from build123d import *

# Parameters (mm, degrees)
BOSS_EXTRUDE1_DEPTH = 5
FILLET3_R           = 1
FILLET4_R           = 1
FILLET5_R           = 4


with BuildPart() as part:
    # Sketch1 → Boss-Extrude1 (new body)
    with BuildSketch(Plane.XY):
        Polygon((0, 5), (0, 19.982808697), (0, 24.6), (0, 29.8), (6.8, 29.8), (6.8, 26.8), (4.8, 26.8), (4.8, 24.6), (10, 24.6), (10, 21.2), (4.8, 21.2), (4.8, 19.6), (20, 19.6), (20, 5), (20, 0), (15, 0), (15, 5), (11.5, 5), (11.5, 8), (12.6, 8), (12.6, 10.3), (11.5, 10.3), (11.5, 15), (8.5, 15), (8.5, 10.3), (7.4, 10.3), (7.4, 8), (8.5, 8), (8.5, 5), (5, 5), (5, 0), (0, 0), align=None)
    extrude(amount=BOSS_EXTRUDE1_DEPTH)

    # Fillet3
    fillet3_edges = [part.edges().sort_by_distance(p)[0] for p in [
        (10, 21.2, 2.5),
        (20, 19.6, 2.5),
    ]]
    fillet(fillet3_edges, radius=FILLET3_R)

    # Fillet4
    fillet4_edges = [part.edges().sort_by_distance(p)[0] for p in [
        (6.8, 29.8, 2.5),
        (6.8, 26.8, 2.5),
        (10, 24.6, 2.5),
    ]]
    fillet(fillet4_edges, radius=FILLET4_R)

    # Fillet5
    fillet5_edges = [part.edges().sort_by_distance(p)[0] for p in [
        (0, 29.8, 2.5),
    ]]
    fillet(fillet5_edges, radius=FILLET5_R)


solid = part.part
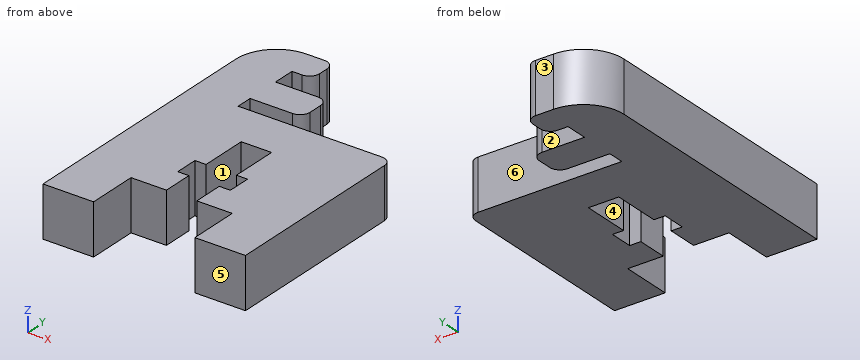
Source: CAD feature listing. Evaluate the final solid. Frame: model axes, mm. Face numbers are marked on the shaded views. A direction names the side the tool comes from. Round coordinates to 2 decimals unless told otherwise and drop trailing zeros. Write each loop counter-clockwise with the first axis right and the second up, starting at its lowest first coordinate (ties: lowest second). Pieces come first, ordered by that corner, then holes. Notation, with made-up numbers: M 74,-15.75 L 84,-15.75 A26 ccw 84,8.25 Z; hole C 46.5,24 d10. An arc over 180 degrees is marked long. One line per item, written item: value. Start each with the question number.
Item 1: Section query A-A (y = 3.5). Return the cut outline in (x, z).
Item 2: Section query C-C (x = 11). Return the cut outline in (y, z).
Item 3: Section query D-D (y = 11). Return the cut outline in (x, z).
Item 4: Mould query, pull axis Y, two halves, no side actions, for the marked faces 4, 5 and 6. Classes: pulls with the +Y half, pulls with the -Y half, needs draft (parallel to the pull), parting line crosses it, or undercut.
Item 5: Pin query (flat end, axial travel): pin 1 (1.8 mm diameter, centred on x = 7.5, z = 1.5, fed in from -Y); pin 2 (1.3 mm diameter, centred on y = 20, z = 1.5, fed in from +X); pin 3 (1.1 mm diameter, centred on y = 22.5, z = 2.5, fed in from +X). Return the tip coordinate at first contact, or that it passes through.
Item 6: Ray query, L1, parallel to X at y = 2, z = 1; L2, parallel to X at y = 9, z = 0.65; L3, parallel to Y at x = 8.25, z = 0.5. Return the intervals inside material, ascending. Write a range as from..to.
Item 7: Set-up query: the marked faces 1, 2 and 3. Return all of +Z, -Z, +X, -X, +Y, -Y with unobstructed straight access to the full face (end or side cutting, diameter ignored); none if empty.
Result set:
1. outline: M 0,0 L 5,0 L 5,5 L 0,5 Z; M 15,0 L 20,0 L 20,5 L 15,5 Z
2. outline: M 15,0 L 19.6,0 L 19.6,5 L 15,5 Z
3. outline: M 0,0 L 8.5,0 L 8.5,5 L 0,5 Z; M 11.5,0 L 20,0 L 20,5 L 11.5,5 Z
4. face 4: needs draft
4. face 5: pulls with the -Y half
4. face 6: undercut
5. pin 1: stops at y = 5
5. pin 2: stops at x = 19.66
5. pin 3: stops at x = 10
6. L1: x = 0..5, 15..20
6. L2: x = 0..7.4, 12.6..20
6. L3: y = 5..8, 10.3..19.6, 21.2..24.6
7. face 1: +Z, -Z, -Y
7. face 2: +Z, -Z, +X
7. face 3: +Z, -Z, +X, -X, +Y
